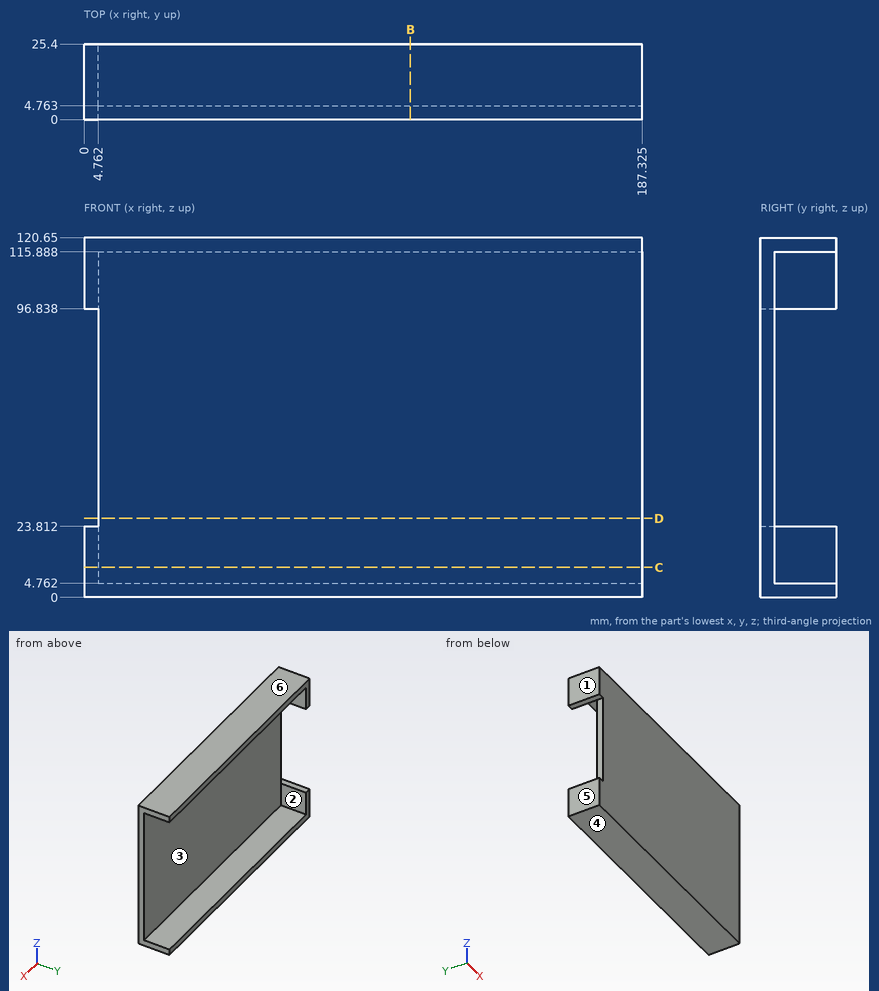
Geometry: see drawing. Coordinates: mm, zero at the bounding-box minimum. A direction names the side the tool comes from. Coordinates: 2 decimals unless noted, no trailing zeros. Loops run counter-clockwise (first coordinate to the right, second up) from the corner with the lowest first, then second, coordinate; pieces in that order, holes last. Notation, with made-up numbers: M 68,1.5 L 123,1.5 A34 ccw 123,38.5 Z; hole C -2.75,-40 d10. An arc over 180 degrees is marked long. Put each result on its own line as item: value. Start each with the question number.
1) Ray query, L1, parallel to Z at x = 25.5, y = 7.25; L2, parallel to Y at x = 59, z = 27.5. Return the intervals inside material, ascending. Write a range as from..to.
2) Pull-direction query (Z, two-part tool) for the marked faces 3, 4, 5 and 6; classes: pulls with the +Z half, pulls with the -Z half, needs draft (parallel to the pull), parting line crosses it, or undercut.
3) Reachability of the marked faces 1 and 2 from +Z, -Z, +X, -X, +Y, -Y: full face, straight path, thin tool, end or side. Return the list, or none.
4) Contact query for flat-ended pins moving along their axis: pin 1 Ø5 at (y, z) = (2.5, 73.5) entering from -X; pin 2 Ø3 at (x, z) = (154.5, 52.5) entering from +Y; pin 3 Ø9.5 at (y, z) = (12, 10) entering from +X. Output: stop coordinate, or through.
5) Cut plane C-C on z = 10. Return the cut outline in (x, y) (1 decimal).
6) Cut plane D-D on z = 26.5. Return the cut outline in (x, y) (1 decimal).
7) Cut plane B-B on x = 109.5. Return the cut outline in (y, z).
The answers:
1. L1: z = 0..4.76, 115.89..120.65
1. L2: y = 0..4.76
2. face 3: undercut
2. face 4: pulls with the -Z half
2. face 5: needs draft
2. face 6: pulls with the +Z half
3. face 1: +Z, -Z, -X, +Y, -Y
3. face 2: +X, +Y
4. pin 1: stops at x = 4.76
4. pin 2: stops at y = 4.76
4. pin 3: stops at x = 4.76
5. outline: M 0,0 L 187.3,0 L 187.3,4.8 L 4.8,4.8 L 4.8,25.4 L 0,25.4 Z
6. outline: M 4.8,0 L 187.3,0 L 187.3,4.8 L 4.8,4.8 Z
7. outline: M 0,0 L 25.4,0 L 25.4,4.76 L 4.76,4.76 L 4.76,115.89 L 25.4,115.89 L 25.4,120.65 L 0,120.65 Z
